from build123d import *

# Parameters (mm, degrees)
BOSS_EXTRUDE1_DEPTH = 25
SHELL1_T            = -7.5
SKETCH3_R           = 3
CUT_EXTRUDE1_DEPTH  = 30
SKETCH4_R           = 2.5
CUT_EXTRUDE2_DEPTH  = 10


with BuildPart() as part:
    # Sketch2 → Boss-Extrude1 (new body)
    with BuildSketch(Plane(origin=(0, 0, 0), x_dir=(1, 0, 0), z_dir=(0, 1, 0))):
        Polygon((10, -35), (42, -15), (42, 0), (0, 0), (0, -35), align=None)
    extrude(amount=BOSS_EXTRUDE1_DEPTH)

    # Shell1
    shell1_openings = [part.faces().sort_by_distance(p)[0] for p in [
        (42, 12.5, 7.5),
        (26, 12.5, 25),
        (5, 12.5, 35),
    ]]
    offset(amount=SHELL1_T, openings=shell1_openings, kind=Kind.INTERSECTION)

    # Sketch3 → Cut-Extrude1 (cut)
    with BuildSketch(Plane(origin=(7.5, 0, 0), x_dir=(0, 0, -1), z_dir=(1, 0, 0))):
        with Locations((-28.75, 12.5)):
            Circle(SKETCH3_R)
        with Locations((-13.75, 12.5)):
            Circle(SKETCH3_R)
    extrude(amount=-CUT_EXTRUDE1_DEPTH, mode=Mode.SUBTRACT)

    # Sketch4 → Cut-Extrude2 (cut)
    with BuildSketch(Plane.XY.offset(7.5)):
        with Locations((17.25, 12.5)):
            Circle(SKETCH4_R)
        with Locations((32.25, 12.5)):
            Circle(SKETCH4_R)
    extrude(amount=-CUT_EXTRUDE2_DEPTH, mode=Mode.SUBTRACT)


solid = part.part
Can you work these out from the model? Positions are in its coordinate system, mm. A direction names the side the tool comes from. Give positions to 0.01 mm unless a question says otherwise; leave off trailing zeros. Loops run counter-clockwise (first coordinate to the right, second up) from the corner with the lowest first, then second, coordinate; pieces in that order, holes last. Notation, with made-up numbers: M -3,-2 L 32,-2 A28 cw 32,26 Z; hole C -8.5,36 d8. An arc over 180 degrees is marked long. One line per item, written item: value. Start each with the question number.
1) If I drill on line 1 (Y direction, x = 32.25, z = 5); line 2 (Y direction, x = 38, z = 15); line 3 (X direction, y = 13, z = 10.5), over which ranges is the centre line in solid material (lowest first)? Write a range as [from, to].
2) On a 3-axis mill with a long thin cutter (end or side, diameter ignored), from which of +Z, -Z, +X, -X, +Y, -Y can I reach the whole of each face in a straight line? I mean faces 4 (the face through (21, 17.5, 18)), 5 (the face through (42, 12, 6)). Say none if no direction works.
3) Thinking about a two-plate mould opening in X: for faces 1 (the face through (26, 4, 25)), 2 (the face through (31.71, 10.06, 3.8)), 3 (the face through (0, 12, 17)), which applies, +X half, -X half, draft (parallel to the pull), parting line (faces both ways), or undercut?
4) If we section it at A-A, the plane z = 28.75: Write out the boundary of the cut face in (x, y).
5) If we section it at B-B, the plane z = 6: Write out the boundary of the cut face in (x, y).
6) I'm going to push flat-ended pins straight in: pin 1 (5.5 mm diameter, centred on y = 12.5, z = 13.75, fed in from +X); pin 2 (6 mm diameter, centred on x = 32.25, y = 12.5, fed in from +Z); pin 3 (2 mm diameter, centred on y = 7.5, z = 23.5, fed in from +X); pin 4 (6 mm diameter, centred on y = 19, z = 27, fed in from +X). Where does each tip first touch, or does it pass through?
7) If we section it at C-C, the plane x = 32.25: Write out the boundary of the cut face in (y, z).
8) If we section it at D-D, the plane y = 19.5: Write out the boundary of the cut face in (x, z), and give its area (3 significant figures).
Completed:
1. line 1: y = [0, 10], [15, 25]
1. line 2: y = [0, 7.5], [17.5, 25]
1. line 3: x = [0, 7.5]
2. face 4: +Z, +X
2. face 5: +Z, -Z, +X, +Y, -Y
3. face 1: +X half
3. face 2: undercut
3. face 3: -X half
4. outline: M 0,0 L 20,0 L 20,7.5 L 7.5,7.5 L 7.5,9.5 L 0,9.5 Z; M 0,15.5 L 7.5,15.5 L 7.5,17.5 L 20,17.5 L 20,25 L 0,25 Z
5. outline: M 0,0 L 42,0 L 42,25 L 0,25 Z; hole C 17.25,12.5 d5; hole C 32.25,12.5 d5
6. pin 1: passes through
6. pin 2: stops at z = 7.5
6. pin 3: stops at x = 30
6. pin 4: stops at x = 27.6
7. outline: M 0,0 L 10,0 L 10,7.5 L 7.5,7.5 L 7.5,21.09 L 0,21.09 Z; M 15,0 L 25,0 L 25,21.09 L 17.5,21.09 L 17.5,7.5 L 15,7.5 Z
8. outline: M 0,0 L 42,0 L 42,15 L 10,35 L 0,35 Z
8. area: 1,150 mm^2
